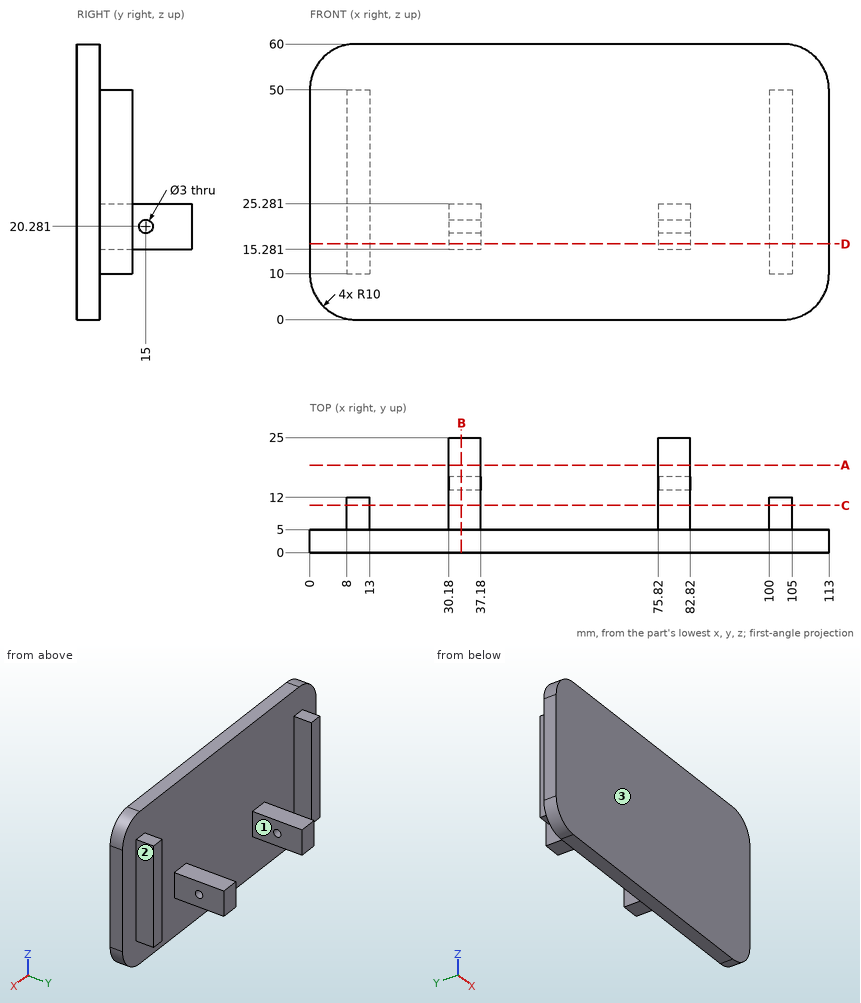
Study the drawing (mm; zero at the part's minimum x, y, z) and answer. Coordinates: 2 decimals unless noted, no trailing zeros. Write each loop counter-clockwise with the first axis right and the second up, starting at its lowest first coordinate (ties: lowest second). Pieces come first, ordered by that corner, then holes.
Q1. A cutting plane is placed at B-B, the plane x = 33. Give the vertices of the cut face in (y, z), then the cut area to 3 significant figures.
Q2. Find the intervals of material crossed by line 1 (X direction, y = 12.75, z = 17); line 2 (Y direction, x = 28.5, z = 30); line 3 (Z direction, x = 34.5, y = 23.75), in increasing order.
Q3. Determine the mould class of the marked faces 1, 2 and 3 for opening direction X: released by +X, released by -X, zero draft, split by the parting line, or undercut.
Q4. A cutting plane is placed at A-A, the plane y = 19. Give the vertices of the cut face in (x, z).
Q5. A cutting plane is placed at D-D, the plane z = 16.5. Give the vertices of the cut face in (x, y), then the cut area to 3 significant figures.
Q6. A cutting plane is placed at C-C, the plane y = 10.25. Give the vertices of the cut face in (x, z).
Q7. Each of these flat-tipped pins is pushed along its axis until it touches: pin 1 Ø10 at (x, z) = (21, 16) entering from +Y; pin 2 Ø3 at (y, z) = (10, 8) entering from -X; pin 3 Ø5.5 at (y, z) = (9.5, 33) entering from -X; pin 4 Ø4 at (x, y) = (11, 10) entering from -Z. Where does it stop, or does it pass through?
Findings below:
1. outline: (0, 0) - (5, 0) - (5, 15.28) - (25, 15.28) - (25, 25.28) - (5, 25.28) - (5, 60) - (0, 60) - close; hole circle Ø3 at (15, 20.28)
1. area: 493 mm2
2. line 1: x = 30.18 to 37.18, 75.82 to 82.82
2. line 2: y = 0 to 5
2. line 3: z = 15.28 to 25.28
3. face 1: undercut
3. face 2: released by +X
3. face 3: zero draft
4. outline: (30.18, 15.28) - (37.18, 15.28) - (37.18, 25.28) - (30.18, 25.28) - close; (75.82, 15.28) - (82.82, 15.28) - (82.82, 25.28) - (75.82, 25.28) - close
5. outline: (0, 0) - (113, 0) - (113, 5) - (105, 5) - (105, 12) - (100, 12) - (100, 5) - (82.82, 5) - (82.82, 25) - (75.82, 25) - (75.82, 5) - (37.18, 5) - (37.18, 25) - (30.18, 25) - (30.18, 5) - (13, 5) - (13, 12) - (8, 12) - (8, 5) - (0, 5) - close
5. area: 915 mm2
6. outline: (8, 10) - (13, 10) - (13, 50) - (8, 50) - close; (30.18, 15.28) - (37.18, 15.28) - (37.18, 25.28) - (30.18, 25.28) - close; (75.82, 15.28) - (82.82, 15.28) - (82.82, 25.28) - (75.82, 25.28) - close; (100, 10) - (105, 10) - (105, 50) - (100, 50) - close
7. pin 1: stops at y = 5
7. pin 2: passes through
7. pin 3: stops at x = 8
7. pin 4: stops at z = 10
